from build123d import *

# Parameters (mm, degrees)
SKETCH1_W           = 78.74
SKETCH1_H           = 19.05
BOSS_EXTRUDE1_DEPTH = 5.08
SKETCH2_W           = 25.4
SKETCH2_H           = 5.08
CUT_EXTRUDE1_DEPTH  = 41.823142028
SKETCH3_W           = 19.05
SKETCH3_H           = 5.08
BOSS_EXTRUDE2_DEPTH = 95.25
SKETCH4_R           = 2.032
CUT_EXTRUDE2_DEPTH  = 5.08


with BuildPart() as part:
    # Sketch1 → Boss-Extrude1 (new body)
    with BuildSketch(Plane(origin=(0, 0, 0), x_dir=(1, 0, 0), z_dir=(0, 1, 0))):
        Rectangle(SKETCH1_W, SKETCH1_H)
    extrude(amount=BOSS_EXTRUDE1_DEPTH)

    # Sketch2 → Cut-Extrude1 (cut, through all)
    with BuildSketch(Plane(origin=(0, 5.08, 0), x_dir=(1, 0, 0), z_dir=(0, 1, 0))):
        Rectangle(SKETCH2_W, SKETCH2_H)
    extrude(amount=-CUT_EXTRUDE1_DEPTH, mode=Mode.SUBTRACT)

    # Sketch3 → Boss-Extrude2 (add)
    with BuildSketch(Plane(origin=(39.37, 0, 0), x_dir=(0, 0, -1), z_dir=(1, 0, 0))):
        with Locations((0, 2.54)):
            Rectangle(SKETCH3_W, SKETCH3_H)
    extrude(amount=BOSS_EXTRUDE2_DEPTH)

    # Sketch4 → Cut-Extrude2 (cut)
    with BuildSketch(Plane.XZ):
        with Locations(Location((125.585488771, 0, 0), (0, 0, 270))):
            Circle(SKETCH4_R)
    extrude(amount=-CUT_EXTRUDE2_DEPTH, mode=Mode.SUBTRACT)


solid = part.part
Source: CAD feature listing. Evaluate the final solid. Frame: model axes, mm. A direction names the side the tool comes from. Give positions to 0.01 mm unless a question says otherwise; leave off trailing zeros. Loops run counter-clockwise (first coordinate to the right, second up) from the corner with the lowest first, then second, coordinate; pieces in that order, holes last. Notation, with made-up numbers: (-21.75, -28.5) -> (20.25, -28.5) arc R7 cw to (20.25, -15.5) -> close; hole circle Ø6 at (68, 46). An arc over 180 degrees is marked (long way). Use a Markdown table: item, result. Add a question column.
1) Reachability of faces 4 (the face through (46, 3, 9.525)), 5 (the face through (0, 3, -2.54)) from +Z, -Z, +X, -X, +Y, -Y: full face, straight path, thin tool, end or side. Return the list, or none.
2) Line query: line 1 along X through (y, z) = (1.55, 0); line 2 along Z through (x, y) = (11, 1.45) (3 decimals); line 3 along X through (y, z) = (3.55, -1). Output: solid intervals per line, ascending. Write a range as [from, to].
3) First-contact query: pin 1 (1 mm diameter, centred on x = 52.5, z = 2, fed in from -Y). Flat tip, straight axial feed; report the tip coordinate or a pass-through.
4) Section query A-A, the plane z = 0. Return the cut outline in (x, y).
5) Section query B-B, the plane y = 4.2. Return the cut outline in (x, z) (3 decimals), then the cut area to 3 significant figures.
6) Pull-direction query (X, two-part tool) for faces 1 (the face through (12.7, 3, 0)), 2 (the face through (46, 5.08, 0)), 3 (the face through (134.62, 3, 0)); classes: +X half, -X half, draft (parallel to the pull), parting line (faces both ways), or undercut.
Numbers:
| question | item | result |
|---|---|---|
| 1 | face 4 | +Z, +X, -X, +Y, -Y |
| 1 | face 5 | +Y, -Y |
| 2 | line 1 | x = [-39.37, -12.7], [12.7, 123.55], [127.62, 134.62] |
| 2 | line 2 | z = [-9.525, -2.54], [2.54, 9.525] |
| 2 | line 3 | x = [-39.37, -12.7], [12.7, 123.82], [127.35, 134.62] |
| 3 | pin 1 | stops at y = 0 |
| 4 | outline | (-39.37, 0) -> (-12.7, 0) -> (-12.7, 5.08) -> (-39.37, 5.08) -> close; (12.7, 0) -> (123.55, 0) -> (123.55, 5.08) -> (12.7, 5.08) -> close; (127.62, 0) -> (134.62, 0) -> (134.62, 5.08) -> (127.62, 5.08) -> close |
| 5 | outline | (-39.37, -9.525) -> (134.62, -9.525) -> (134.62, 9.525) -> (-39.37, 9.525) -> close; hole (-12.7, -2.54) -> (12.7, -2.54) -> (12.7, 2.54) -> (-12.7, 2.54) -> close; hole circle Ø4.064 at (125.585, 0) |
| 5 | area | 3,170 mm2 |
| 6 | face 1 | undercut |
| 6 | face 2 | draft |
| 6 | face 3 | +X half |
